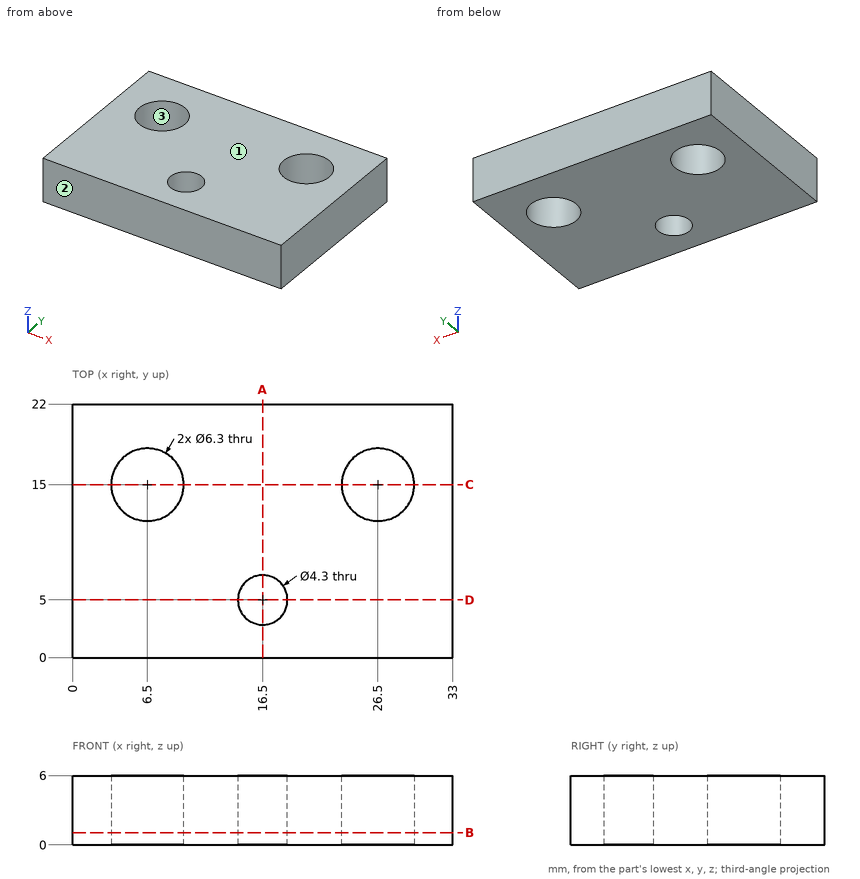
Here's the drawing with two shaded views (mm, measured from the low corner). I have some questions. Round coordinates to 2 decimals unless told otherwise and drop trailing zeros. Write each loop counter-clockwise with the first axis right and the second up, starting at its lowest first coordinate (ties: lowest second). Pieces come first, ordered by that corner, then holes.
(1) Suppose I cut it at B-B on z = 1.05. Write out the boundary of the cut face in (x, y).
Findings below:
outline: (0, 0) - (33, 0) - (33, 22) - (0, 22) - close; hole circle Ø6.3 at (6.5, 15); hole circle Ø4.3 at (16.5, 5); hole circle Ø6.3 at (26.5, 15)
(2) Thinking about a two-plate mould opening in Y: for the marked faces 1, 2 and 3, which applies, +Y half, -Y half, draft (parallel to the pull), parting line (faces both ways), or undercut?
Findings below:
face 1: draft
face 2: -Y half
face 3: undercut
(3) If I drill on probe 1 along X at (y, z) = (13.75, 3.4); probe 2 along Y at (x, z) = (6.5, 2.75); probe 3 along Y at (x, z) = (16.5, 1.9), over which ranges is the centre line in solid material (lowest first)?
Findings below:
probe 1: x = 0 to 3.61, 9.39 to 23.61, 29.39 to 33
probe 2: y = 0 to 11.85, 18.15 to 22
probe 3: y = 0 to 2.85, 7.15 to 22
(4) Suppose I cut it at C-C on y = 15. Write out the boundary of the cut face in (x, z), and give its area (3 significant figures).
Findings below:
outline: (0, 0) - (3.35, 0) - (3.35, 6) - (0, 6) - close; (9.65, 0) - (23.35, 0) - (23.35, 6) - (9.65, 6) - close; (29.65, 0) - (33, 0) - (33, 6) - (29.65, 6) - close
area: 122 mm2
(5) Suppose I cut it at D-D on y = 5. Write out the boundary of the cut face in (x, z).
Findings below:
outline: (0, 0) - (14.35, 0) - (14.35, 6) - (0, 6) - close; (18.65, 0) - (33, 0) - (33, 6) - (18.65, 6) - close
(6) Suppose I cut it at A-A on x = 16.5. Write out the boundary of the cut face in (y, z), and give its area (3 significant figures).
Findings below:
outline: (0, 0) - (2.85, 0) - (2.85, 6) - (0, 6) - close; (7.15, 0) - (22, 0) - (22, 6) - (7.15, 6) - close
area: 106 mm2
(7) For pin 1 (3 mm diameter, centred on x = 4.5, y = 11, fed in from -Z), with a flat end and sliding along its axis, tell me the tip position at first contact or that it passes through.
Findings below:
pin 1: stops at z = 0
